from build123d import *

# Parameters (mm, degrees)
PLINTH_BLOCK_DEPTH                  = 72
SKETCH2_W                           = 142
SKETCH2_H                           = 193.6
HOLLOW_BAY_AND_FRONT_VOID_DEPTH     = 34.65
SKETCH3_W                           = 152.6
SKETCH3_H                           = 2.4
DISH_SUPPORT_RIBS_DEPTH             = 68.8
SKETCH4_R                           = 64
DISH_FLOOR_THICKENING_DEPTH         = 4.8
SKETCH5_R                           = 12
ROD_SOCKET_BOSS_DEPTH               = 48.8
SKETCH6_W                           = 22
SKETCH6_H                           = 54
MORTISE_BLOCK_DEPTH                 = 8.8
SKETCH7_W                           = 10
SKETCH7_H                           = 13.3
END_PANEL_SCREW_BOSSES_DEPTH        = 40.8
SKETCH8_R                           = 6.2
ROD_SOCKET_DEPTH                    = 3.5
SKETCH9_W                           = 16.4
SKETCH9_H                           = 48.4
COLUMN_MORTISE_DEPTH                = 3.5
SKETCH10_R                          = 1
SEAT_PIN_HOLES_DEPTH                = 2.5
SKETCH11_W                          = 16
SKETCH11_H                          = 41
SPILL_DRAIN_CHANNEL_DEPTH           = 1.5
SKETCH12_R                          = 35.75
SKETCH12_R_2                        = 34.25
BOTTLE_POSITION_MARKER_GROOVE_DEPTH = 0.8
CABLE_GROMMET_HOLES_DEPTH           = 195.123671921
CABLE_GROMMET_HOLES_DEPTH_BACK      = 195.123671921
SKETCH13_R                          = 9
SKETCH13_R_2                        = 6
SKETCH14_W                          = 72
SKETCH14_H                          = 28
PI_SIDE_PORT_NOTCH_AND_VENTS_DEPTH  = 2.6
SKETCH15_R                          = 1.3
END_PANEL_SCREW_HOLES_DEPTH         = 6.5


with BuildPart() as part:
    # Sketch1 → Plinth_block (new body)
    with BuildSketch(Plane.XY):
        with BuildLine():
            Line((-138, -100), (138, -100))
            ThreePointArc((138, -100), (146.485281374, -96.485281374), (150, -88))
            Line((150, -88), (150, 88))
            ThreePointArc((150, 88), (146.485281374, 96.485281374), (138, 100))
            Line((138, 100), (-138, 100))
            ThreePointArc((-138, 100), (-146.485281374, 96.485281374), (-150, 88))
            Line((-150, 88), (-150, -88))
            ThreePointArc((-150, -88), (-146.485281374, -96.485281374), (-138, -100))
        make_face()
    extrude(amount=PLINTH_BLOCK_DEPTH)

    # Sketch2 → Hollow_bay_and_front_void (cut, symmetric)
    with BuildSketch(Plane.XY.offset(34.15)):
        with Locations((-80, 0)):
            Rectangle(SKETCH2_W, SKETCH2_H)
        with BuildLine():
            Line((3.2, -96.8), (137.8, -96.8))
            ThreePointArc((137.8, -96.8), (144.163961031, -94.163961031), (146.8, -87.8))
            Line((146.8, -87.8), (146.8, 87.8))
            ThreePointArc((146.8, 87.8), (144.163961031, 94.163961031), (137.8, 96.8))
            Line((137.8, 96.8), (3.2, 96.8))
            ThreePointArc((3.2, 96.8), (-3.163961031, 94.163961031), (-5.8, 87.8))
            Line((-5.8, 87.8), (-5.8, -87.8))
            ThreePointArc((-5.8, -87.8), (-3.163961031, -94.163961031), (3.2, -96.8))
        make_face()
    extrude(amount=HOLLOW_BAY_AND_FRONT_VOID_DEPTH, both=True, mode=Mode.SUBTRACT)

    # Sketch3 → Dish_support_ribs (add)
    with BuildSketch(Plane.XY):
        with Locations((70.5, 40)):
            Rectangle(SKETCH3_W, SKETCH3_H)
        with Locations((70.5, -40)):
            Rectangle(SKETCH3_W, SKETCH3_H)
    extrude(amount=DISH_SUPPORT_RIBS_DEPTH)

    # Sketch4 → Dish_floor_thickening (add)
    with BuildSketch(Plane.XY.offset(64)):
        with Locations((70, 0)):
            Circle(SKETCH4_R)
    extrude(amount=DISH_FLOOR_THICKENING_DEPTH)

    # Sketch5 → Rod_socket_boss (add)
    with BuildSketch(Plane.XY.offset(20)):
        Circle(SKETCH5_R)
    extrude(amount=ROD_SOCKET_BOSS_DEPTH)

    # Sketch6 → Mortise_block (add)
    with BuildSketch(Plane.XY.offset(60)):
        with Locations((-84, 0)):
            Rectangle(SKETCH6_W, SKETCH6_H)
    extrude(amount=MORTISE_BLOCK_DEPTH)

    # Sketch7 → End_panel_screw_bosses (add)
    with BuildSketch(Plane.XY.offset(28)):
        with Locations((-145, 90.65)):
            Rectangle(SKETCH7_W, SKETCH7_H)
        with Locations((-145, -90.65)):
            Rectangle(SKETCH7_W, SKETCH7_H)
    extrude(amount=END_PANEL_SCREW_BOSSES_DEPTH)

    # Sketch8 → Rod_socket (cut, symmetric)
    with BuildSketch(Plane.XY.offset(69.5)):
        Circle(SKETCH8_R)
    extrude(amount=ROD_SOCKET_DEPTH, both=True, mode=Mode.SUBTRACT)

    # Sketch9 → Column_mortise (cut, symmetric)
    with BuildSketch(Plane.XY.offset(69.5)):
        with Locations((-84, 0)):
            Rectangle(SKETCH9_W, SKETCH9_H)
    extrude(amount=COLUMN_MORTISE_DEPTH, both=True, mode=Mode.SUBTRACT)

    # Sketch10 → Seat_pin_holes (cut, symmetric)
    with BuildSketch(Plane.XY.offset(70.5)):
        with Locations((70, 50)):
            Circle(SKETCH10_R)
        with Locations((26.698729811, -25)):
            Circle(SKETCH10_R)
        with Locations((113.301270189, -25)):
            Circle(SKETCH10_R)
    extrude(amount=SEAT_PIN_HOLES_DEPTH, both=True, mode=Mode.SUBTRACT)

    # Sketch11 → Spill_drain_channel (cut, symmetric)
    with BuildSketch(Plane.XY.offset(71.5)):
        with Locations((70, -80.5)):
            Rectangle(SKETCH11_W, SKETCH11_H)
    extrude(amount=SPILL_DRAIN_CHANNEL_DEPTH, both=True, mode=Mode.SUBTRACT)

    # Sketch12 → Bottle_position_marker_groove (cut, symmetric)
    with BuildSketch(Plane.XY.offset(72.2)):
        with Locations((-112, -62)):
            Circle(SKETCH12_R)
        with Locations((-112, -62)):
            Circle(SKETCH12_R_2, mode=Mode.SUBTRACT)
    extrude(amount=BOTTLE_POSITION_MARKER_GROOVE_DEPTH, both=True, mode=Mode.SUBTRACT)

    # Sketch13 → Cable_grommet_holes (cut, two sides: drawn at the far end of the back side and taken through both)
    with BuildSketch(Plane.XY.offset(-CABLE_GROMMET_HOLES_DEPTH_BACK)):
        with Locations((-30, 60)):
            Circle(SKETCH13_R)
        with Locations((-110, 0)):
            Circle(SKETCH13_R_2)
        with Locations((-112, -18)):
            Circle(SKETCH13_R_2)
    extrude(amount=CABLE_GROMMET_HOLES_DEPTH + CABLE_GROMMET_HOLES_DEPTH_BACK, mode=Mode.SUBTRACT)

    # Sketch14 → Pi_side_port_notch_and_vents (cut, symmetric)
    with BuildSketch(Plane(origin=(0, 98.4, 0), x_dir=(1, 0, 0), z_dir=(0, 1, 0))):
        with Locations((-92, -13)):
            Rectangle(SKETCH14_W, SKETCH14_H)
        with BuildLine():
            Line((-138, -50), (-129, -50))
            ThreePointArc((-129, -50), (-127.585786438, -50.585786438), (-127, -52))
            Line((-127, -52), (-127, -56))
            ThreePointArc((-127, -56), (-127.585786438, -57.414213562), (-129, -58))
            Line((-129, -58), (-138, -58))
            ThreePointArc((-138, -58), (-139.414213562, -57.414213562), (-140, -56))
            Line((-140, -56), (-140, -52))
            ThreePointArc((-140, -52), (-139.414213562, -50.585786438), (-138, -50))
        make_face()
        with BuildLine():
            Line((-118, -50), (-109, -50))
            ThreePointArc((-109, -50), (-107.585786438, -50.585786438), (-107, -52))
            Line((-107, -52), (-107, -56))
            ThreePointArc((-107, -56), (-107.585786438, -57.414213562), (-109, -58))
            Line((-109, -58), (-118, -58))
            ThreePointArc((-118, -58), (-119.414213562, -57.414213562), (-120, -56))
            Line((-120, -56), (-120, -52))
            ThreePointArc((-120, -52), (-119.414213562, -50.585786438), (-118, -50))
        make_face()
        with BuildLine():
            Line((-98, -50), (-89, -50))
            ThreePointArc((-89, -50), (-87.585786438, -50.585786438), (-87, -52))
            Line((-87, -52), (-87, -56))
            ThreePointArc((-87, -56), (-87.585786438, -57.414213562), (-89, -58))
            Line((-89, -58), (-98, -58))
            ThreePointArc((-98, -58), (-99.414213562, -57.414213562), (-100, -56))
            Line((-100, -56), (-100, -52))
            ThreePointArc((-100, -52), (-99.414213562, -50.585786438), (-98, -50))
        make_face()
        with BuildLine():
            Line((-78, -50), (-69, -50))
            ThreePointArc((-69, -50), (-67.585786438, -50.585786438), (-67, -52))
            Line((-67, -52), (-67, -56))
            ThreePointArc((-67, -56), (-67.585786438, -57.414213562), (-69, -58))
            Line((-69, -58), (-78, -58))
            ThreePointArc((-78, -58), (-79.414213562, -57.414213562), (-80, -56))
            Line((-80, -56), (-80, -52))
            ThreePointArc((-80, -52), (-79.414213562, -50.585786438), (-78, -50))
        make_face()
        with BuildLine():
            Line((-58, -50), (-49, -50))
            ThreePointArc((-49, -50), (-47.585786438, -50.585786438), (-47, -52))
            Line((-47, -52), (-47, -56))
            ThreePointArc((-47, -56), (-47.585786438, -57.414213562), (-49, -58))
            Line((-49, -58), (-58, -58))
            ThreePointArc((-58, -58), (-59.414213562, -57.414213562), (-60, -56))
            Line((-60, -56), (-60, -52))
            ThreePointArc((-60, -52), (-59.414213562, -50.585786438), (-58, -50))
        make_face()
        with BuildLine():
            Line((-38, -50), (-29, -50))
            ThreePointArc((-29, -50), (-27.585786438, -50.585786438), (-27, -52))
            Line((-27, -52), (-27, -56))
            ThreePointArc((-27, -56), (-27.585786438, -57.414213562), (-29, -58))
            Line((-29, -58), (-38, -58))
            ThreePointArc((-38, -58), (-39.414213562, -57.414213562), (-40, -56))
            Line((-40, -56), (-40, -52))
            ThreePointArc((-40, -52), (-39.414213562, -50.585786438), (-38, -50))
        make_face()
    extrude(amount=PI_SIDE_PORT_NOTCH_AND_VENTS_DEPTH, both=True, mode=Mode.SUBTRACT)

    # Sketch15 → End_panel_screw_holes (cut, symmetric)
    with BuildSketch(Plane(origin=(-144.5, 0, 0), x_dir=(0, 0, -1), z_dir=(1, 0, 0))):
        with Locations((-35, 90)):
            Circle(SKETCH15_R)
        with Locations((-35, -90)):
            Circle(SKETCH15_R)
    extrude(amount=END_PANEL_SCREW_HOLES_DEPTH, both=True, mode=Mode.SUBTRACT)


solid = part.part
Here's how the part is built. I have some questions about the finished solid (model axes, mm). A direction names the side the tool comes from. Give positions to 0.01 mm unless a question says otherwise; leave off trailing zeros. Order: outer loops, then holes, each group sorted by start corner. A loop starts at its lowest first (then second) coordinate and runs counter-clockwise, first axis right, second up. Notation, with made-up numbers: M 14.5,79.25 L 21.5,79.25 A17 cw 21.5,90.25 Z; hole C 54.25,-12 d10. An arc over 180 degrees is marked long. Answer as a JSON object with one key per item and string values. Group by question number.
1) On a 3-axis mill with a long thin cutter (end or side, diameter ignored), from which of +Z, -Z, +X, -X, +Y, -Y can I reach the whole of each face in a straight line? I mean faces 1 (the flat face through (4, 28, 68.8)), 2 (the flat face through (-145, 84, 48)), 3 (the flat face through (-75.8, 0, 69)). Say none if no direction works.
2) Please list where these lines run through material, in increasing order: L1, parallel to Y at x = 23.5, z = 32; L2, parallel to X at y = -53, z = 48; L3, parallel to Y at x = -30, z = 70. Write a range as [from, to].
3) Suppose I cut it at C-C, the plane y = 60. Write out the boundary of the cut face in (x, z).
4) Suppose I cut it at B-B, the plane z = 13.5. Count the separate pieces of the cut face and the enclosed holes in it, plus the area to 3 significant figures.
5) Suppose I cut it at A-A, the plane x = -52. Write out the boundary of the cut face in (y, z), plus the area to 3 significant figures.
6) Suppose I cut it at D-D, the plane x = -84. Write out the boundary of the cut face in (y, z).
7) I'm going to push flat-ended pins straight in: pin 1 Ø1 at (x, y) = (27, -25) entering from +Z; pin 2 Ø12 at (x, y) = (-89.5, 7.5) entering from -Z; pin 3 Ø10 at (y, z) = (68.5, 19) entering from -X. Where does each tip first touch, or does it pass through?
8) We'd pull the mould along X, two halves only. Please class faces 4 (the cylindrical face through (133.997, -0.584, 66.366)), 5 (the flat face through (-84, 27, 64)), 6 (the cylindrical face through (146.39, -96.58, 35.5)): pulls with the +X half, pulls with the -X half, needs draft (parallel to the pull), parting line crosses it, or undercut.
Results found:
{
 "1": {"face 1": "-Z", "face 2": "-Z, -X", "face 3": "+Z"},
 "2": {"L1": "[-100, -96.8], [-41.2, -38.8], [38.8, 41.2], [96.8, 100]", "L2": "[-9, -5.8], [146.8, 150]", "L3": "[-100, 51], [69, 100]"},
 "3": {"outline": "M -150,68.8 L -39,68.8 L -39,72 L -150,72 Z; M -21,68.8 L -9,68.8 L -9,0 L -5.8,0 L -5.8,68.8 L 47.73,68.8 L 47.73,64 L 92.27,64 L 92.27,68.8 L 146.8,68.8 L 146.8,0 L 150,0 L 150,72 L -21,72 Z"},
 "4": {"separate pieces": "2", "enclosed holes": "3", "area": "3,630 mm²"},
 "5": {"outline": "M -100,0 L -96.8,0 L -96.8,68.8 L 96.8,68.8 L 96.8,58 L 100,58 L 100,72 L -100,72 Z; M 96.8,0 L 100,0 L 100,50 L 96.8,50 Z", "area": "1,050 mm²"},
 "6": {"outline": "M -100,0 L -96.8,0 L -96.8,68.8 L -27,68.8 L -27,60 L 27,60 L 27,68.8 L 96.8,68.8 L 96.8,27 L 100,27 L 100,72 L 24.2,72 L 24.2,66 L -24.2,66 L -24.2,72 L -39.77,72 L -39.77,71.4 L -42.28,71.4 L -42.28,72 L -81.72,72 L -81.72,71.4 L -84.23,71.4 L -84.23,72 L -100,72 Z"},
 "7": {"pin 1": "z = 68", "pin 2": "z = 60", "pin 3": "x = -9"},
 "8": {"face 4": "undercut", "face 5": "needs draft", "face 6": "pulls with the +X half"}
}
